Could you check a few things on this drawing? It's one solid part, dimensions in mm from its lowest x, y, z. Give positions to 0.01 mm unless a question says otherwise; leave off trailing zeros. Loops run counter-clockwise (first coordinate to the right, second up) from the corner with the lowest first, then second, coordinate; pieces in that order, holes last. Notation, with made-up numbers: (15.25, -26.75) - (32.25, -26.75) arc R24 ccw to (32.25, -11.75) - close; hole circle Ø2 at (44.25, 46). An arc over 180 degrees is marked (long way). Answer as a JSON object with one key per item and string values.
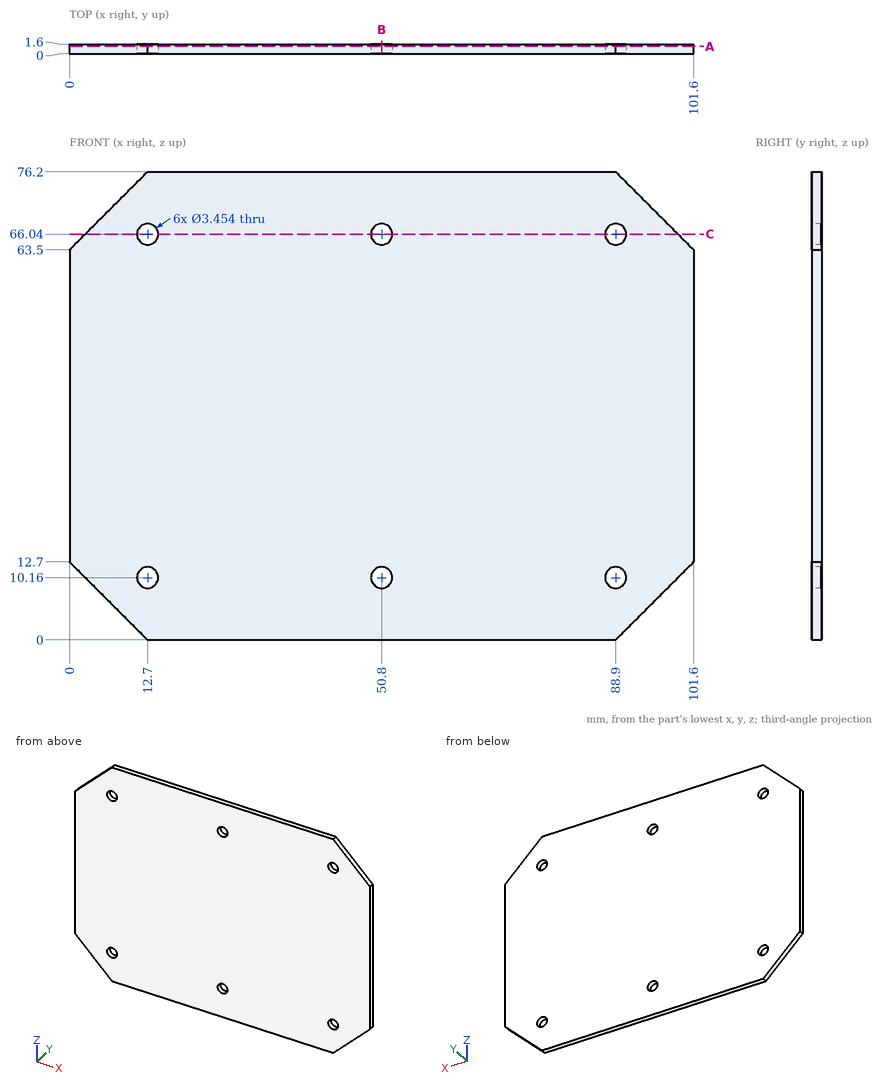
1) Imagine slicing it at C-C on z = 66.04. Write out the boundary of the cut face in (x, y), and give its area (3 significant figures).
Check sheet entries:
{"outline": "(2.54, 0) - (10.97, 0) - (10.97, 1.6) - (2.54, 1.6) - close; (14.43, 0) - (49.07, 0) - (49.07, 1.6) - (14.43, 1.6) - close; (52.53, 0) - (87.17, 0) - (87.17, 1.6) - (52.53, 1.6) - close; (90.63, 0) - (99.06, 0) - (99.06, 1.6) - (90.63, 1.6) - close", "area": "138 mm2"}
2) I'm going to push a flat-ended pin straight in: P1, Ø3, axis at x = 12.7, z = 66.04, coming from the -Y side. Where does the tip first touch, or does it pass through?
Check sheet entries:
{"P1": "through"}
3) Imagine slicing it at A-A on y = 1.2. Write out the boundary of the cut face in (x, z) (1 decimal).
Check sheet entries:
{"outline": "(0, 12.7) - (12.7, 0) - (88.9, 0) - (101.6, 12.7) - (101.6, 63.5) - (88.9, 76.2) - (12.7, 76.2) - (0, 63.5) - close; hole circle Ø3.5 at (12.7, 10.2); hole circle Ø3.5 at (12.7, 66); hole circle Ø3.5 at (50.8, 10.2); hole circle Ø3.5 at (50.8, 66); hole circle Ø3.5 at (88.9, 10.2); hole circle Ø3.5 at (88.9, 66)"}
4) Imagine slicing it at B-B on x = 50.8. Write out the boundary of the cut face in (y, z).
Check sheet entries:
{"outline": "(0, 0) - (1.6, 0) - (1.6, 8.43) - (0, 8.43) - close; (0, 11.89) - (1.6, 11.89) - (1.6, 64.31) - (0, 64.31) - close; (0, 67.77) - (1.6, 67.77) - (1.6, 76.2) - (0, 76.2) - close"}
5) I need wall thicknesses on L1, parallel to Z at x = 50.8, y = 0.45; L2, parallel to X at y = 0.45, z = 66.04 (1 decimal); L3, parallel to Z at x = 52, y = 1.35. Which ranges of each line are inside material? Lowest first, please.
Check sheet entries:
{"L1": "0 to 8.43, 11.89 to 64.31, 67.77 to 76.2", "L2": "2.5 to 11, 14.4 to 49.1, 52.5 to 87.2, 90.6 to 99.1", "L3": "0 to 8.92, 11.4 to 64.8, 67.28 to 76.2"}
